Here's how the part is built. I have some questions about the finished solid (model axes, mm). Face numbers are marked on the shaded views. A direction names the side the tool comes from. Give positions to 0.01 mm unless a question says otherwise; leave off trailing zeros. Write each loop counter-clockwise with the first axis right and the second up, starting at its lowest first coordinate (ties: lowest second). Pieces come first, ordered by that corner, then holes. Notation, with made-up numbers: M 5,22 L 16,22 A19 cw 16,42 Z; hole C 16.25,-23.75 d6. An arc over 180 degrees is marked long. Use one line per item in the form item = value. Start each with the question number.
from build123d import *

# Parameters (mm, degrees)
SKETCH1_W                = 2
SKETCH1_H                = 31.74
BOSS_EXTRUDE1_DEPTH      = 40
BOSS_EXTRUDE1_2_DEPTH    = 40
SKETCH2_W                = 37
SKETCH2_H                = 31.74
BOSS_EXTRUDE3_DEPTH      = 2
SKETCH8_W                = 37
SKETCH8_H                = 3
BOSS_EXTRUDE4_DEPTH      = 70
SKETCH12_R               = 18
BOSS_EXTRUDE6_DEPTH      = 74
BOSS_EXTRUDE6_DEPTH_BACK = 3
SKETCH18_R               = 16.1
CUT_EXTRUDE2_DEPTH       = 75
SKETCH19_R               = 3.5
CUT_EXTRUDE3_DEPTH       = 74
SKETCH20_R               = 6.36
SKETCH20_R_2             = 1.78
SKETCH20_R_3             = 2.03
CUT_EXTRUDE4_DEPTH       = 3.24
CUT_EXTRUDE4_DEPTH_BACK  = 35.76


with BuildPart() as part:
    # Sketch1 → Boss-Extrude1 (new body)
    with BuildSketch(Plane(origin=(0, 0, 0), x_dir=(1, 0, 0), z_dir=(0, 1, 0))):
        with Locations((-2.074327578, -14.662349727)):
            Rectangle(SKETCH1_W, SKETCH1_H)
    extrude(amount=BOSS_EXTRUDE1_DEPTH)



with BuildPart() as body_2:
    # Sketch1 → Boss-Extrude1 2 (new body)
    with BuildSketch(Plane(origin=(0, 0, 0), x_dir=(1, 0, 0), z_dir=(0, 1, 0))):
        with Locations((28.453672422, -14.662349727)):
            Rectangle(SKETCH1_W, SKETCH1_H)
    extrude(amount=BOSS_EXTRUDE1_2_DEPTH)


with BuildPart() as part_1:
    add(part.part)

    add(body_2.part)  # Boss-Extrude3 merges body 2
    # Sketch2 → Boss-Extrude3 (add)
    with BuildSketch(Plane(origin=(0, 40, 0), x_dir=(1, 0, 0), z_dir=(0, 1, 0))):
        with Locations((13.193672422, -14.662349727)):
            Rectangle(SKETCH2_W, SKETCH2_H)
    extrude(amount=-BOSS_EXTRUDE3_DEPTH)

    # Sketch8 → Boss-Extrude4 (add)
    with BuildSketch(Plane(origin=(0, 40, 0), x_dir=(1, 0, 0), z_dir=(0, 1, 0))):
        with Locations((13.193672422, -14.662349727)):
            Rectangle(SKETCH8_W, SKETCH8_H)
    extrude(amount=BOSS_EXTRUDE4_DEPTH)

    # Sketch12 → Boss-Extrude6 (add, two sides)
    with BuildSketch(Plane(origin=(0, 0, 13.162349727), x_dir=(-1, 0, 0), z_dir=(0, 0, -1))) as boss_extrude6_sk:
        with Locations((-13.193672422, 110)):
            Circle(SKETCH12_R)
    extrude(amount=BOSS_EXTRUDE6_DEPTH)
    extrude(boss_extrude6_sk.sketch, amount=-BOSS_EXTRUDE6_DEPTH_BACK)

    # Sketch18 → Cut-Extrude2 (cut)
    with BuildSketch(Plane(origin=(0, 0, -60.837650273), x_dir=(-1, 0, 0), z_dir=(0, 0, -1))):
        with Locations((-13.193672422, 110)):
            Circle(SKETCH18_R)
    extrude(amount=-CUT_EXTRUDE2_DEPTH, mode=Mode.SUBTRACT)

    # Sketch19 → Cut-Extrude3 (cut)
    with BuildSketch(Plane(origin=(0, 0, 14.162349727), x_dir=(-1, 0, 0), z_dir=(0, 0, -1))):
        with Locations((-13.193672422, 110)):
            Circle(SKETCH19_R)
    extrude(amount=-CUT_EXTRUDE3_DEPTH, mode=Mode.SUBTRACT)

    # Sketch20 → Cut-Extrude4 (cut, two sides)
    with BuildSketch(Plane(origin=(29.453672422, 0, 0), x_dir=(0, 0, -1), z_dir=(1, 0, 0))) as cut_extrude4_sk:
        with Locations((-17.842349727, 16.779878139)):
            Circle(SKETCH20_R)
        with Locations((-17.842349727, 26.558878139)):
            Circle(SKETCH20_R_2)
        with Locations((-17.842349727, 7.000878139)):
            Circle(SKETCH20_R_2)
        with Locations((-27.367349727, 16.779878139)):
            Circle(SKETCH20_R_3)
        with Locations((-8.317349727, 16.779878139)):
            Circle(SKETCH20_R_3)
    extrude(amount=CUT_EXTRUDE4_DEPTH, mode=Mode.SUBTRACT)
    extrude(cut_extrude4_sk.sketch, amount=-CUT_EXTRUDE4_DEPTH_BACK, mode=Mode.SUBTRACT)


solid = part_1.part
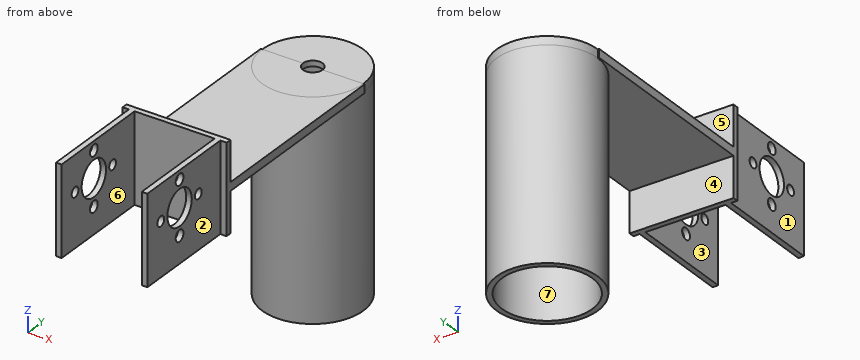
1) Will these pins go through, and if not, where does the flat tip stop? P1, Ø6, axis at x = 0, z = -48.5, coming from the +Y side; P2, Ø5.5, axis at y = 7, z = 17.84, coming from the -X side; P3, Ø3, axis at y = 16.78, z = 27.37, coming from the +X side; P4, Ø8.5, axis at x = 19, z = 16.5, coming from the -Y side.
2) Suppose I cut it at A-A, the plane y = 111.5. List the corners of the cut face in (x, z) for me, and give its area (3 significant figures).
3) Please list where these lines run through material, in increasing order: line 1 (Y direction, x = 24, z = 3.5); line 2 (Y direction, x = 17, z = 1.5); line 3 (Y direction, x = 22.5, z = -42.5).
4) Suppose I cut it at B-B, the plane z = -18.5. List the corners of the cut face in (x, y) for me.
5) On a 3-axis mill with a long thin cutter (end or side, diameter ignored), from which of +Z, -Z, +X, -X, +Y, -Y can I reach the whole of each face in a straight line? I mean the marked faces 1, 2, 3 and 4. Say none if no direction works.
6) Suppose I cut it at D-D, the plane y = 57. List the corners of the cut face in (x, z) for me.
7) Thinking about a two-plate mould opening in Y: for the marked faces 5, 6 and 7, which applies, released by +Y, released by -Y, zero draft, split by the parting line, or undercut?
8) Suppose I cut it at C-C, the plane x = 4. List the corners of the cut face in (y, z) for me, and give its area (3 significant figures).
Checks:
q1.P1 = 124.84
q1.P2 = -3.07
q1.P3 = through
q1.P4 = 38
q2.outline = M -4.74,-60.84 L -2.84,-60.84 L -2.84,14.16 L 10.03,14.16 L 10.03,16.16 L -4.74,16.16 Z; M 16.36,14.16 L 29.22,14.16 L 29.22,-60.84 L 31.13,-60.84 L 31.13,16.16 L 16.36,16.16 Z
q2.area = 345 mm^2
q3.line_1 = 38 to 40, 95.6 to 98.07, 121.93 to 124.4
q3.line_2 = 38 to 40, 92.41 to 94.36, 125.64 to 127.59
q3.line_3 = 94.59 to 96.86, 123.14 to 125.41
q4.outline = C 13.19,110 d36; hole C 13.19,110 d32.2
q5.face_1 = +Z, -Z, -X, -Y
q5.face_2 = +Z, -Z, +X, -Y
q5.face_3 = +Z, -Z, -Y
q5.face_4 = -Z, +X, -X
q6.outline = M -5.31,13.16 L 31.69,13.16 L 31.69,16.16 L -5.31,16.16 Z
q7.face_5 = released by +Y
q7.face_6 = zero draft
q7.face_7 = undercut
q8.outline = M 38,-1.21 L 40,-1.21 L 40,13.16 L 94.52,13.16 L 94.52,-60.84 L 96.78,-60.84 L 96.78,14.16 L 123.22,14.16 L 123.22,-60.84 L 125.48,-60.84 L 125.48,16.16 L 40,16.16 L 40,30.53 L 38,30.53 Z
q8.area = 628 mm^2
